Build history of the part. All positions in model axes, mm. A direction names the side the tool comes from. Give positions to 0.01 mm unless a question says otherwise; leave off trailing zeros. Order: outer loops, then holes, each group sorted by start corner. A loop starts at its lowest first (then second) coordinate and runs counter-clockwise, first axis right, second up. Notation, with made-up numbers: (-33, 60) - (24, 60) arc R11 ccw to (24, 76) - close; hole circle Ø9 at (70, -24.5). An arc over 180 degrees is marked (long way). Use a Markdown table: item, result.
from build123d import *

# Parameters (mm, degrees)
BOSS_EXTRUDE1_DEPTH = 6.35
SKETCH2_R           = 2.54
CUT_EXTRUDE1_DEPTH  = 6.35
FILLET1_R           = 9.525


with BuildPart() as part:
    # Sketch1 → Boss-Extrude1 (new body)
    with BuildSketch(Plane(origin=(0, 0, 0), x_dir=(1, 0, 0), z_dir=(0, 1, 0))):
        with BuildLine():
            Line((0, 0), (0, -76.2))
            Line((0, -76.2), (17.766321776, -114.3))
            Line((17.766321776, -114.3), (35.031485119, -106.249122114))
            Line((35.031485119, -106.249122114), (19.05, -71.976716677))
            Line((19.05, -71.976716677), (19.05, -69.85))
            ThreePointArc((19.05, -69.85), (32.069103576, -38.419103576), (63.5, -25.4))
            Line((63.5, -25.4), (101.6, -25.4))
            Line((101.6, -25.4), (101.6, 0))
            Line((101.6, 0), (0, 0))
        make_face()
    extrude(amount=BOSS_EXTRUDE1_DEPTH)

    # Sketch2 → Cut-Extrude1 (cut)
    with BuildSketch(Plane(origin=(0, 6.35, 0), x_dir=(1, 0, 0), z_dir=(0, 1, 0))):
        with Locations(Location((12.7, -12.7, 0), (0, 0, 270))):
            Circle(SKETCH2_R)
        with Locations(Location((38.1, -12.7, 0), (0, 0, 270))):
            Circle(SKETCH2_R)
        with Locations(Location((63.5, -12.7, 0), (0, 0, 270))):
            Circle(SKETCH2_R)
        with Locations(Location((88.9, -12.7, 0), (0, 0, 270))):
            Circle(SKETCH2_R)
        with Locations((114.3, -12.7)):
            Circle(SKETCH2_R)
        with Locations((139.7, -12.7)):
            Circle(SKETCH2_R)
        with Locations(Location((12.7, -38.1, 0), (0, 0, 270))):
            Circle(SKETCH2_R)
    extrude(amount=-CUT_EXTRUDE1_DEPTH, mode=Mode.SUBTRACT)

    # Fillet1
    fillet1_edges = [part.edges().sort_by_distance(p)[0] for p in [
        (17.766321776, 3.175, 114.3),
        (35.031485119, 3.175, 106.249122114),
    ]]
    fillet(fillet1_edges, radius=FILLET1_R - 0.0001)  # a hair under: the kernel refuses the full size


solid = part.part
1) Slice it at B-B (z = 12.7). Write the cut outline in (x, y), and give its area (3 significant figures).
Computed:
| item | result |
|---|---|
| outline | (0, 0) - (10.16, 0) - (10.16, 6.35) - (0, 6.35) - close; (15.24, 0) - (35.56, 0) - (35.56, 6.35) - (15.24, 6.35) - close; (40.64, 0) - (60.96, 0) - (60.96, 6.35) - (40.64, 6.35) - close; (66.04, 0) - (86.36, 0) - (86.36, 6.35) - (66.04, 6.35) - close; (91.44, 0) - (101.6, 0) - (101.6, 6.35) - (91.44, 6.35) - close |
| area | 516 mm² |
2) Slice it at C-C (x = 38.1). Write the cut outline in (y, z), and give its area (3 significant figures).
Computed:
| item | result |
|---|---|
| outline | (0, 0) - (6.35, 0) - (6.35, 10.16) - (0, 10.16) - close; (0, 15.24) - (6.35, 15.24) - (6.35, 33.37) - (0, 33.37) - close |
| area | 180 mm² |
3) Slice it at A-A (y = 2). State how many separate pieces and enclosed holes the cut face has, and give its area (3 significant figures).
Computed:
| item | result |
|---|---|
| separate pieces | 1 |
| enclosed holes | 5 |
| area | 4,550 mm² |
4) Tool access for faces 4 (the flat face through (52, 3, 0)), 5 (the cylindrical face through (31.725, 3.131, 38.767)), 6 (the flat face through (82, 3, 25.4)): list every direction of +Z, -Z, +X, -X, +Y, -Y with a clear straight run to the whole face (end or side of a thin tool).
Computed:
| item | result |
|---|---|
| face 4 | -Z, +X, -X, +Y, -Y |
| face 5 | +X, +Y, -Y |
| face 6 | +Z, +X, +Y, -Y |
5) Pin check, flat tips, straight feed: P1, Ø1.5, axis at x = 36.5, y = 1.5, coming from the +Z side; P2, Ø3, axis at x = 38.1, z = 12.7, coming from the -Y side; P3, Ø0.6, axis at y = 5, z = 71, coming from the +X side; P4, Ø2, axis at x = 66, y = 4, coming from the +Z side. Stop position of each tip, or through.
Computed:
| item | result |
|---|---|
| P1 | stops at z = 35.13 |
| P2 | passes through |
| P3 | stops at x = 19.05 |
| P4 | stops at z = 25.4 |
6) Wall check: line 1 (X direction, y = 4, z = 12.7); line 2 (Z direction, x = 95.5, y = 6); line 3 (X direction, y = 4.75, z = 12). Give the ranges that are in metal, low to high. Write a range as from..to.
Computed:
| item | result |
|---|---|
| line 1 | x = 0..10.16, 15.24..35.56, 40.64..60.96, 66.04..86.36, 91.44..101.6 |
| line 2 | z = 0..25.4 |
| line 3 | x = 0..10.26, 15.14..35.66, 40.54..61.06, 65.94..86.46, 91.34..101.6 |
7) Two-plate mould, pull along Z, no slides. Class faces 1 (the cylindrical face through (15.22, 3.22, 12.37)), 2 (the cylindrical face through (19.017, 3.219, 110.556)), 3 (the flat face through (39, 6.35, 30)): +Z half, -Z half, draft (parallel to the pull), parting line (faces both ways), or undercut.
Computed:
| item | result |
|---|---|
| face 1 | undercut |
| face 2 | +Z half |
| face 3 | draft |
8) Slice it at D-D (z = 38.1). Write the cut outline in (x, y).
Computed:
| item | result |
|---|---|
| outline | (0, 0) - (10.16, 0) - (10.16, 6.35) - (0, 6.35) - close; (15.24, 0) - (32.39, 0) - (32.39, 6.35) - (15.24, 6.35) - close |
